Job drawing, mm, ordinate dimensions from the low corner. One solid piece. Round coordinates to 2 decimals unless told otherwise and drop trailing zeros. Loops run counter-clockwise (first coordinate to the right, second up) from the corner with the lowest first, then second, coordinate; pieces in that order, holes last.
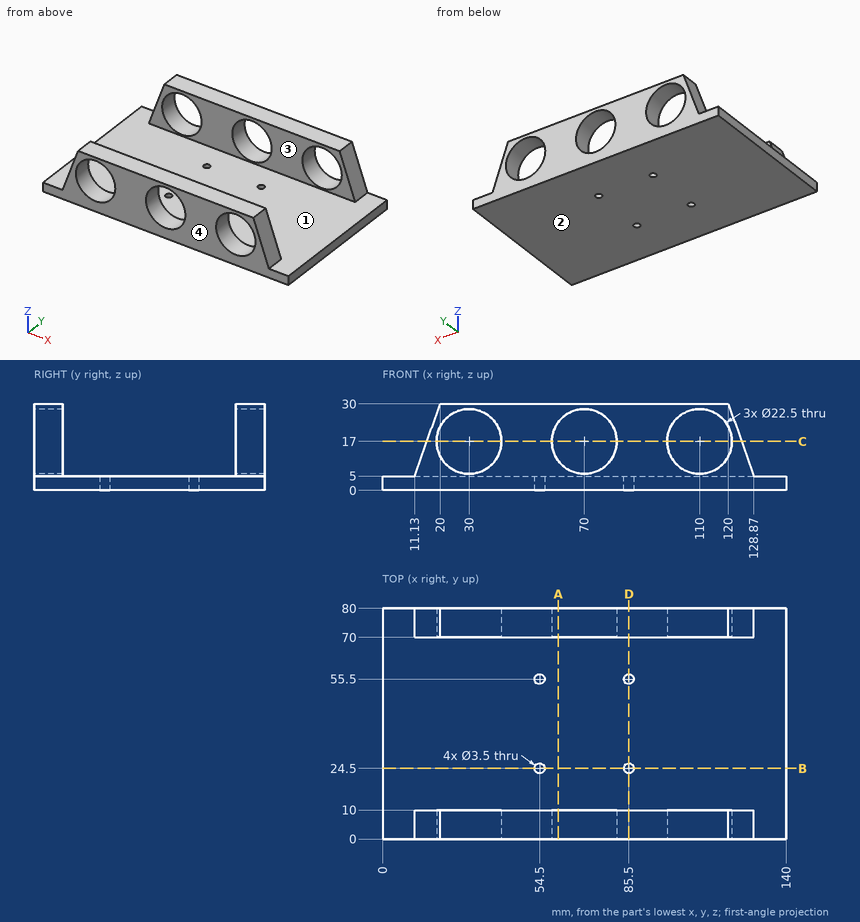
(1) Slice it at A-A on x = 61. List the corners of the cut face in (y, z).
Responses:
outline: (0, 0) - (80, 0) - (80, 10.25) - (70, 10.25) - (70, 5) - (10, 5) - (10, 10.25) - (0, 10.25) - close; (0, 23.75) - (10, 23.75) - (10, 30) - (0, 30) - close; (70, 23.75) - (80, 23.75) - (80, 30) - (70, 30) - close
(2) Slice it at C-C on z = 17. Count the separate pieces of the cut face and the enclosed holes in it.
Responses:
separate pieces: 8
enclosed holes: 0
(3) Pin check, flat tips, straight feed: P1, Ø8, axis at x = 33.5, y = 27.5, coming from the +Z side; P2, Ø8, axis at x = 27.5, y = 49.5, coming from the -Z side. Stop position of each tip, or through.
Responses:
P1: stops at z = 5
P2: stops at z = 0
(4) Probe line 1 (Y direction, x = 54.5, z = 3.6); line 2 (Y direction, x = 82.5, z = 28); line 3 (X direction, y = 78.25, z = 17). List the from-to ranges inside material, lowest first.
Responses:
line 1: y = 0 to 22.75, 26.25 to 53.75, 57.25 to 80
line 2: y = 0 to 10, 70 to 80
line 3: x = 15.39 to 18.75, 41.25 to 58.75, 81.25 to 98.75, 121.25 to 124.61
(5) Slice it at D-D on x = 85.5. List the corners of the cut face in (y, z), plus the area to 3 significant figures.
Responses:
outline: (0, 0) - (22.75, 0) - (22.75, 5) - (10, 5) - (10, 30) - (0, 30) - close; (26.25, 0) - (53.75, 0) - (53.75, 5) - (26.25, 5) - close; (57.25, 0) - (80, 0) - (80, 30) - (70, 30) - (70, 5) - (57.25, 5) - close
area: 865 mm2
(6) Slice it at B-B on y = 24.5. List the corners of the cut face in (x, z).
Responses:
outline: (0, 0) - (52.75, 0) - (52.75, 5) - (0, 5) - close; (56.25, 0) - (83.75, 0) - (83.75, 5) - (56.25, 5) - close; (87.25, 0) - (140, 0) - (140, 5) - (87.25, 5) - close
(7) Pull direction Y, two halves, no side cores. Call the marked faces 1, 2, 3 and 4: +Y half, -Y half, draft (parallel to the pull), parting line (faces both ways), or undercut.
Responses:
face 1: undercut
face 2: draft
face 3: undercut
face 4: -Y half
